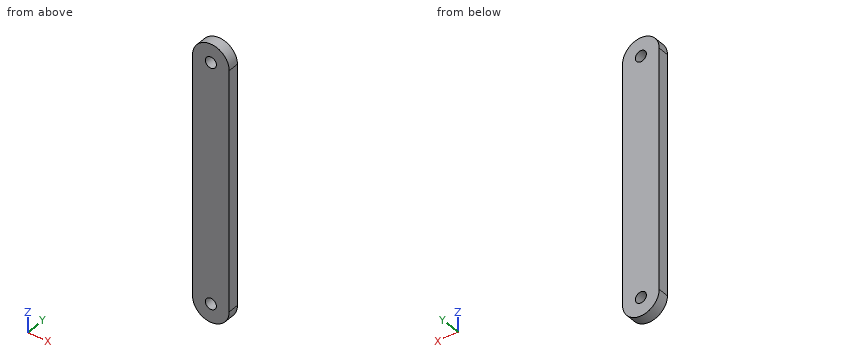
Autodesk Fusion 360 part; units mm, degrees
sketch "Sketch1" plane through (0, 0, 0) normal (0, 1, 0) x (1, 0, 0)
  line L0 (5, 32.5) -> (-5, 32.5)
  line L1 (-5, 32.5) -> (-5, -32.5)
  line L2 (-5, -32.5) -> (5, -32.5)
  line L3 (5, -32.5) -> (5, 32.5)
  line L4 (5, 32.5) -> (-5, -32.5) construction
  line L5 (-5, 32.5) -> (5, -32.5) construction
  arc A0 (5, 32.5) -> (-5, 32.5) centre (0, 32.5) ccw
  line L6 (-5, 0) -> (5, 0) construction
  circle A1 centre (0, 32.5) radius 1.5
  arc A2 (-5, -32.5) -> (5, -32.5) centre (0, -32.5) ccw
  circle A3 centre (0, -32.5) radius 1.5
  dimension "d1" = 10
  dimension "d2" = 65
  dimension "d3" = 3
extrude "Extrude1" add sketch "Sketch1" along normal blind 3 contours L0 L1 L2 L3 A1 A3 | L0 A0 A1 | L2 A2 A3
CAD build for the part. Positions are in the model's coordinates, mm. Coordinates: 2 decimals unless noted, no trailing zeros. Loops run counter-clockwise (first coordinate to the right, second up) from the corner with the lowest first, then second, coordinate; pieces in that order, holes last. Notation, with made-up numbers: (-39.5, 31) - (0.5, 31) arc R25 cw to (0.5, 62) - close; hole circle Ø2 at (-29.75, 80). An arc over 180 degrees is marked (long way). Write item = value, one per line. Start each with the question number.
Q1. Cut at A-A, the plane x = 0. List the corners of the cut face in (y, z).
Q2. Cut at C-C, the plane x = 3.5. List the corners of the cut face in (y, z).
Q3. Cut at B-B, the plane y = 0.55. List the corners of the cut face in (x, z).
Q4. Drill centre lines: L1, parallel to Z at x = -1.25, y = 2.3; L2, parallel to Z at x = 1, y = 1.15; L3, parallel to X at y = 1.05, z = -32.5. Where is each one in solid material? Low to high.
Computed:
q1.outline = (0, -37.5) - (3, -37.5) - (3, -34) - (0, -34) - close; (0, -31) - (3, -31) - (3, 31) - (0, 31) - close; (0, 34) - (3, 34) - (3, 37.5) - (0, 37.5) - close
q2.outline = (0, -36.07) - (3, -36.07) - (3, 36.07) - (0, 36.07) - close
q3.outline = (-5, -32.5) arc R5 ccw to (5, -32.5) - (5, 32.5) arc R5 ccw to (-5, 32.5) - close; hole circle Ø3 at (0, -32.5); hole circle Ø3 at (0, 32.5)
q4.L1 = -37.34 to -33.33, -31.67 to 31.67, 33.33 to 37.34
q4.L2 = -37.4 to -33.62, -31.38 to 31.38, 33.62 to 37.4
q4.L3 = -5 to -1.5, 1.5 to 5
